from build123d import *

# Parameters (mm, degrees)
F0_R     = 3
F0_R_2   = 8
F1_DEPTH = 5
F2_R     = 12.5
F2_R_2   = 8
F3_DEPTH = 12


with BuildPart() as f1:
    # F0 (on Front) → F1 (new body)
    with BuildSketch(Plane.XZ):
        with BuildLine():
            Line((-21.354157, -13), (21.354157, -13))
            ThreePointArc((21.354157, -13), (0, 25), (-21.354157, -13))
        make_face()
        with Locations((-17, 0)):
            Circle(F0_R, mode=Mode.SUBTRACT)
        Circle(F0_R_2, mode=Mode.SUBTRACT)
        with Locations((17, 0)):
            Circle(F0_R, mode=Mode.SUBTRACT)
    extrude(amount=F1_DEPTH)

    # F2 (on face) → F3 (join)
    with BuildSketch(Plane.XZ.offset(5)):
        Circle(F2_R)
        Circle(F2_R_2, mode=Mode.SUBTRACT)
    extrude(amount=F3_DEPTH)


solid = f1.part
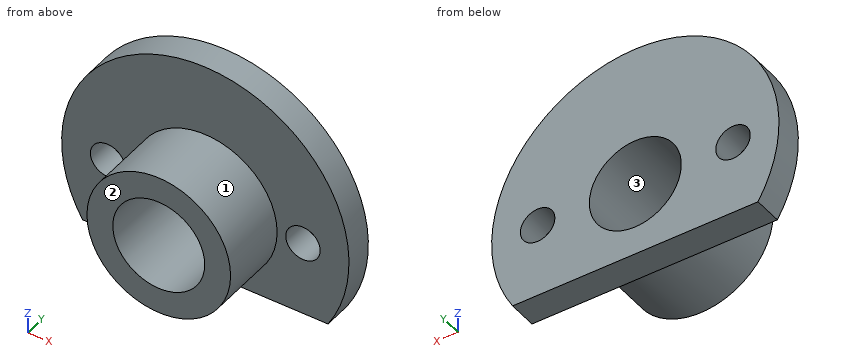
Can you work these out from the model? Positions are in its coordinate system, mm. Face numbers are marked on the shaded views. Give positions to 0.01 mm unless a question says otherwise; leave off trailing zeros. Loops run counter-clockwise (first coordinate to the right, second up) from the corner with the lowest first, then second, coordinate; pieces in that order, holes last. Notation, with made-up numbers: (31, -26.75) - (82, -26.75) arc R19 ccw to (82, 8.25) - close; hole circle Ø4 at (70, -12.75). An arc over 180 degrees is marked (long way). Answer as a JSON object with one key per item and string values.
Q1. Imagine slicing it at D-D on z = 4. Write out the boundary of the cut face in (x, y).
Geometry says:
{"outline": "(-24.68, -5) - (-11.84, -5) - (-11.84, -17) - (-6.93, -17) - (-6.93, 0) - (-24.68, 0) - close; (6.93, -17) - (11.84, -17) - (11.84, -5) - (24.68, -5) - (24.68, 0) - (6.93, 0) - close"}
Q2. If I drill on L1, parallel to Y at x = -13, z = 2.5; L2, parallel to Z at x = 0, y = -8; L3, parallel to X at y = -2.25, z = 4, over which ranges is the centre line in solid material (lowest first)?
Geometry says:
{"L1": "-5 to 0", "L2": "-12.5 to -8, 8 to 12.5", "L3": "-24.68 to -6.93, 6.93 to 24.68"}
Q3. Imagine slicing it at C-C on y = -2.25. Write out the boundary of the cut face in (x, z).
Geometry says:
{"outline": "(-21.35, -13) - (21.35, -13) arc R25 ccw (long way) to start; hole circle Ø6 at (-17, 0); hole circle Ø16 at (0, 0); hole circle Ø6 at (17, 0)"}
Q4. Will these pins go through, and if not, where does the flat tip stop? P1, Ø8, axis at x = -16, y = -5.5, coming from the +Z side; P2, Ø8, axis at x = 17, z = 0, coming from the -Y side; P3, Ø2, axis at x = -15, z = 17, coming from the +Y side; P4, Ø4, axis at y = -5.5, z = -6, coming from the -X side.
Geometry says:
{"P1": "z = 21.91", "P2": "y = -5", "P3": "y = 0", "P4": "x = -24.67"}
Q5. Imagine slicing it at B-B on z = 0. Write out the boundary of the cut face in (x, y), plus the area to 3 significant figures.
Geometry says:
{"outline": "(-25, -5) - (-20, -5) - (-20, 0) - (-25, 0) - close; (-14, -5) - (-12.5, -5) - (-12.5, -17) - (-8, -17) - (-8, 0) - (-14, 0) - close; (8, -17) - (12.5, -17) - (12.5, -5) - (14, -5) - (14, 0) - (8, 0) - close; (20, -5) - (25, -5) - (25, 0) - (20, 0) - close", "area": "218 mm²"}
Q6. Imagine slicing it at A-A on x = 0. Write out the boundary of the cut face in (y, z).
Geometry says:
{"outline": "(-17, -12.5) - (-5, -12.5) - (-5, -13) - (0, -13) - (0, -8) - (-17, -8) - close; (-17, 8) - (0, 8) - (0, 25) - (-5, 25) - (-5, 12.5) - (-17, 12.5) - close"}
Q7. If we mould it in two halves opening along Z, with no side actions, what happens to the marked faces 1, 2 and 3? For each: pulls with the +Z half, pulls with the -Z half, needs draft (parallel to the pull), parting line crosses it, or undercut.
Geometry says:
{"face 1": "parting line crosses it", "face 2": "needs draft", "face 3": "undercut"}
